Could you check a few things on this drawing? It's one solid part, dimensions in mm from its lowest x, y, z. A direction names the side the tool comes from. Give positions to 0.01 mm unless a question says otherwise; leave off trailing zeros. Loops run counter-clockwise (first coordinate to the right, second up) from the corner with the lowest first, then second, coordinate; pieces in that order, holes last.
1. Imagine slicing it at A-A (z = 7.75). List the corners of the cut face in (x, y) for me.
2. Imagine slicing it at B-B (y = 1.8). List the corners of the cut face in (x, z) for me.
3. Imagine slicing it at C-C (x = 10.5). List the corners of the cut face in (y, z) for me.
4. For P1, Ø2, axis at x = 16, y = 1.5, coming from the -Z side, with a flat end and sliding along its axis, tell me the tip position at first contact or that it passes through.
5. I need wall thicknesses on line 1 along X through (y, z) = (1.2, 2); line 2 along X through (y, z) = (3.4, 16.5); line 3 along Z through (x, y) = (17.5, 2). Which ranges of each line are inside material? Lowest first, please.
6. For the marked faces 1 and 2, which set-ups out of +Z, -Z, +X, -X, +Y, -Y let a thin tool reach every point of the face, with its end or its side?
7. Imagine slicing it at D-D (x = 25). List the corners of the cut face in (y, z) for me.
8. Thinking about a two-plate mould opening in X: for the marked faces 3, 4 and 5, which applies, +X half, -X half, draft (parallel to the pull), parting line (faces both ways), or undercut?
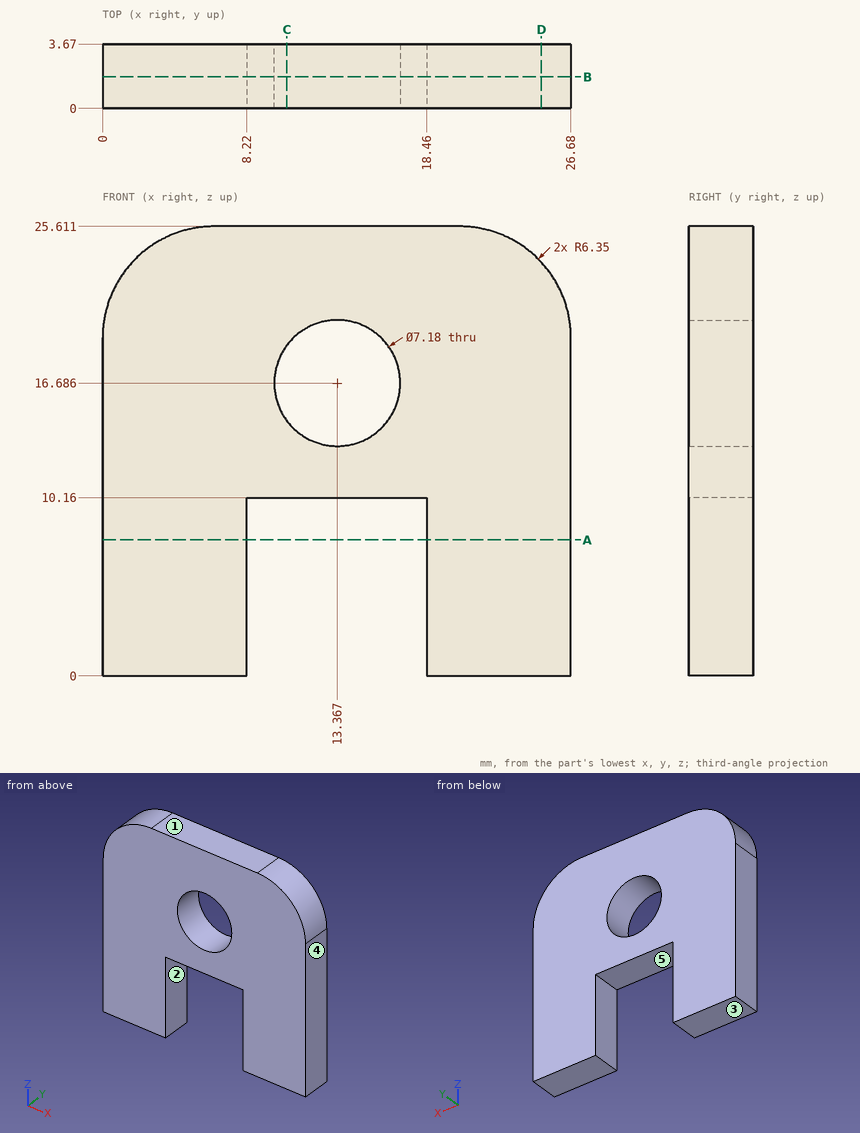
Derived:
1. outline: (0, 0) - (8.22, 0) - (8.22, 3.67) - (0, 3.67) - close; (18.46, 0) - (26.68, 0) - (26.68, 3.67) - (18.46, 3.67) - close
2. outline: (0, 0) - (8.22, 0) - (8.22, 10.16) - (18.46, 10.16) - (18.46, 0) - (26.68, 0) - (26.68, 19.26) arc R6.35 ccw to (20.33, 25.61) - (6.35, 25.61) arc R6.35 ccw to (0, 19.26) - close; hole circle Ø7.18 at (13.37, 16.69)
3. outline: (0, 10.16) - (3.67, 10.16) - (3.67, 14.53) - (0, 14.53) - close; (0, 18.85) - (3.67, 18.85) - (3.67, 25.61) - (0, 25.61) - close
4. P1: stops at z = 10.16
5. line 1: x = 0 to 8.22, 18.46 to 26.68
5. line 2: x = 0 to 9.78, 16.95 to 26.68
5. line 3: z = 10.16 to 25.61
6. face 1: +Z, +X, -X, +Y, -Y
6. face 2: -Z, +Y, -Y
7. outline: (0, 0) - (3.67, 0) - (3.67, 23.56) - (0, 23.56) - close
8. face 3: draft
8. face 4: +X half
8. face 5: undercut
